```python
from build123d import *

# Parameters (mm, degrees)
SKETCH_1_W          = 28.5
SKETCH_1_H          = 21.5
EXTRUDE_1_DEPTH     = 11.2
FILLET_1_R          = 1
SKETCH_3_W          = 14
SKETCH_3_H          = 14
CUT_EXTRUDE_2_DEPTH = 2
SKETCH_4_W          = 15.8
SKETCH_4_H          = 15.8
CUT_EXTRUDE_3_DEPTH = 0.8


with BuildPart() as part:
    # 草图1 → 凸台-拉伸1 (new body)
    with BuildSketch(Plane(origin=(0, 0, 0), x_dir=(1, 0, 0), z_dir=(0, 1, 0))):
        Rectangle(SKETCH_1_W, SKETCH_1_H)
    extrude(amount=EXTRUDE_1_DEPTH)

    # 圆角1
    fillet_1_edges = [part.edges().sort_by_distance(p)[0] for p in [
        (14.25, 5.6, 10.75),
        (-14.25, 5.6, 10.75),
        (-14.25, 5.6, -10.75),
        (14.25, 5.6, -10.75),
    ]]
    fillet(fillet_1_edges, radius=FILLET_1_R)

    # 草图3 → 切除-拉伸2 (cut)
    with BuildSketch(Plane(origin=(0, 11.2, 0), x_dir=(1, 0, 0), z_dir=(0, 1, 0))):
        Rectangle(SKETCH_3_W, SKETCH_3_H)
    extrude(amount=-CUT_EXTRUDE_2_DEPTH, mode=Mode.SUBTRACT)

    # 草图4 → 切除-拉伸3 (cut)
    with BuildSketch(Plane(origin=(0, 11.2, 0), x_dir=(1, 0, 0), z_dir=(0, 1, 0))):
        Rectangle(SKETCH_4_W, SKETCH_4_H)
    extrude(amount=-CUT_EXTRUDE_3_DEPTH, mode=Mode.SUBTRACT)


solid = part.part
```
Input: part model. Units: mm. Frame: model coordinates. A direction names the side the tool comes from. Give positions to 0.01 mm unless a question says otherwise; leave off trailing zeros. Write each loop counter-clockwise with the first axis right and the second up, starting at its lowest first coordinate (ties: lowest second). Pieces come first, ordered by that corner, then holes. Notation, with made-up numbers: (-21, -17) - (3, -17) arc R27 cw to (3, 8) - close; hole circle Ø7 at (-37.5, 69). An arc over 180 degrees is marked (long way). Write item = value, one per line. Start each with the question number.
1. Ray query, L1, parallel to X at y = 9.75, z = 5.25; L2, parallel to Z at x = -6.25, y = 10.5; L3, parallel to Y at x = 0.25, z = 5.25. Return the intervals inside material, ascending.
2. Section query B-B, the plane z = 4. Output: boundary loops of the cut face in (x, y).
3. Access query for faces 5 (the cylindrical face through (13.965, 5.678, -10.449)), 6 (the flat face through (0, 11, -7.9)). Directions: +Z, -Z, +X, -X, +Y, -Y. A direction counts if a zero-diameter tool reaches every point of the face in a straight line with its end or side. Return the directions, or none.
4. Section query A-A, the plane x = -7.5. Output: boundary loops of the cut face in (y, z).
5. First-contact query: pin 1 Ø4 at (x, z) = (8, -1) entering from -Y; pin 2 Ø7 at (x, z) = (2, 0.5) entering from +Y. Flat tips, straight axial feed; report the tip coordinate or a pass-through.
6. Mould query, pull axis X, two halves, no side actions, for faces 1 (the flat face through (14.25, 6, 0)), 2 (the flat face through (7.9, 11, 0)), 3 (the flat face through (0, 6, -10.75)), 4 (the cylindrical face through (-13.965, 5.678, 10.449)). Classes: released by +X, released by -X, zero draft, split by the parting line, or undercut.
7. Section query C-C, the plane x = 2.25. Output: boundary loops of the cut face in (y, z).
Check sheet entries:
q1.L1 = -14.25 to -7, 7 to 14.25
q1.L2 = -10.75 to -7.9, 7.9 to 10.75
q1.L3 = 0 to 9.2
q2.outline = (-14.25, 0) - (14.25, 0) - (14.25, 11.2) - (7.9, 11.2) - (7.9, 10.4) - (7, 10.4) - (7, 9.2) - (-7, 9.2) - (-7, 10.4) - (-7.9, 10.4) - (-7.9, 11.2) - (-14.25, 11.2) - close
q3.face_5 = -Z, +X, +Y, -Y
q3.face_6 = +Y
q4.outline = (0, -10.75) - (11.2, -10.75) - (11.2, -7.9) - (10.4, -7.9) - (10.4, 7.9) - (11.2, 7.9) - (11.2, 10.75) - (0, 10.75) - close
q5.pin_1 = 0
q5.pin_2 = 9.2
q6.face_1 = released by +X
q6.face_2 = undercut
q6.face_3 = zero draft
q6.face_4 = released by -X
q7.outline = (0, -10.75) - (11.2, -10.75) - (11.2, -7.9) - (10.4, -7.9) - (10.4, -7) - (9.2, -7) - (9.2, 7) - (10.4, 7) - (10.4, 7.9) - (11.2, 7.9) - (11.2, 10.75) - (0, 10.75) - close
